Source: CAD feature listing. Evaluate the final solid. Frame: model axes, mm. A direction names the side the tool comes from. Round coordinates to 2 decimals unless told otherwise and drop trailing zeros. Loops run counter-clockwise (first coordinate to the right, second up) from the corner with the lowest first, then second, coordinate; pieces in that order, holes last.
(1) Section B-B, the plane x = -13. Return the cut outline in (y, z), plus the area to 3 significant figures.
(2) Set-up query: faces 1 (the flat face through (-29.5, -1.2, 1.2)), 2 (the flat face through (0, -4, -14)), 3 (the cylindrical face through (67.744, 19.334, -2.539)), 4 (the cylindrical face through (4.51, 6.31, -20.03)), 5 (the cylindrical face through (-27.5, 6.8, 0)). Return all of +Z, -Z, +X, -X, +Y, -Y with unobstructed straight access to the full face (end or side cutting, diameter ignored); none if empty.
(3) Section A-A, the plane x = 41.5. Return the cut outline in (y, z), plus the area to 3 significant figures.
(4) First-contact query: pin 1 Ø2 at (y, z) = (17.5, 0) entering from -X; pin 2 Ø12 at (x, y) = (-11, -5) entering from -Z; pin 3 Ø8 at (x, z) = (-19, -0.5) entering from -Y. Flat tips, straight axial feed; report the tip coordinate or a pass-through.
(5) Mould query, pull axis Z, two halves, no side actions, for faces 6 (the cylindrical face through (3.042, 0.496, -19.074)), 7 (the cylindrical face through (-3.493, 6.645, -0.251)), 8 (the cylindrical face through (3.04, 18.89, -0.89)), 9 (the flat face through (-18, 7, 2)). Classes: pulls with the +Z half, pulls with the -Z half, needs draft (parallel to the pull), parting line crosses it, or undercut.
(6) Material intervals for probe 1 along Y at (x, z) = (-28, 0) (3 decimals); probe 2 along Y at (x, z) = (67.4, 0), sorted ascending.
```python
from build123d import *

# Parameters (mm, degrees)
SKETCH2_R                = 14
BOSS_EXTRUDE1_DEPTH      = 3
SKETCH3_R                = 6
BOSS_EXTRUDE2_DEPTH      = 26.5
BOSS_EXTRUDE3_DEPTH      = 1
BOSS_EXTRUDE4_REACH      = 80.626
BOSS_EXTRUDE4_END_RADIUS = 6
HOLE1_D                  = 39
HOLE1_DEPTH              = 4.45
HOLE2_D                  = 3.3
HOLE2_DEPTH              = 6
HOLE2_TIP                = 0.991420021
HOLE3_D                  = 3.3
HOLE3_DEPTH              = 6
HOLE3_TIP                = 0.991420021
HOLE4_D                  = 3.3
HOLE4_DEPTH              = 6
HOLE4_TIP                = 0.991420021
HOLE5_D                  = 3.3
HOLE5_DEPTH              = 6
HOLE5_TIP                = 0.991420021
HOLE6_D                  = 1.25
HOLE6_DEPTH              = 1.939156082
HOLE6_CSINK_D            = 2.65
HOLE6_CSINK_ANGLE        = 60
HOLE6_TIP                = 0.360843918


with BuildPart() as part:
    # Sketch1 → Revolve1 (revolve)
    with BuildSketch(Plane.XY, mode=Mode.PRIVATE) as revolve1_sk:
        with BuildLine():
            Line((0, 21), (0, 0))
            Line((0, 0), (70, 0))
            Line((70, 0), (70, 21))
            Line((70, 21), (9.25, 21))
            ThreePointArc((9.25, 21), (9.2, 20.98660254), (9.15, 21))
            Line((9.15, 21), (0, 21))
        make_face()
    revolve(revolve1_sk.sketch.rotate(Axis((0, 0, 0), (1, 0, 0)), 270), axis=Axis((0, 0, 0), (1, 0, 0)))

    # Sketch2 → Boss-Extrude1 (add)
    with BuildSketch(Plane.ZY):
        Circle(SKETCH2_R)
    extrude(amount=BOSS_EXTRUDE1_DEPTH)

    # Sketch3 → Boss-Extrude2 (add)
    with BuildSketch(Plane.ZY.offset(3)):
        Circle(SKETCH3_R)
    extrude(amount=BOSS_EXTRUDE2_DEPTH)

    # Sketch4 → Boss-Extrude3 (add)
    with BuildSketch(Plane.ZY.offset(3)):
        with BuildLine():
            Line((0.293916284, -7.616838781), (0.293916284, -5.992796778))
            ThreePointArc((0.293916284, -5.992796778), (0, 6), (-0.293916284, -5.992796778))
            Line((-0.293916284, -5.992796778), (-0.293916284, -7.616838781))
            ThreePointArc((-0.293916284, -7.616838781), (-1.755912185, -7.072113956), (-2.882513969, -5.992796778))
            ThreePointArc((-2.882513969, -5.992796778), (0, 6.65), (2.882513969, -5.992796778))
            ThreePointArc((2.882513969, -5.992796778), (1.821852016, -7.17721696), (0.293916284, -7.616838781))
        make_face()
    extrude(amount=BOSS_EXTRUDE3_DEPTH)

    # Boss-Extrude4: up to this cylinder (the profile starts outside it)
    boss_extrude4_end = Plane(origin=(-17.5, 0, 0), z_dir=(1, 0, 0)) * Cylinder(BOSS_EXTRUDE4_END_RADIUS, 174.252, mode=Mode.PRIVATE)
    # Sketch5 → Boss-Extrude4 (add, up to the surface)
    with BuildSketch(Plane(origin=(0, 8, 0), x_dir=(-1, 0, 0), z_dir=(0, 1, 0)), mode=Mode.PRIVATE) as boss_extrude4_sk1:
        with BuildLine():
            Line((9.5, -2), (25.5, -2))
            ThreePointArc((25.5, -2), (27.5, 0), (25.5, 2))
            Line((25.5, 2), (9.5, 2))
            ThreePointArc((9.5, 2), (7.5, 0), (9.5, -2))
        make_face()
    boss_extrude4_tool1 = extrude(boss_extrude4_sk1.sketch, amount=-BOSS_EXTRUDE4_REACH, mode=Mode.PRIVATE) - boss_extrude4_end
    add(boss_extrude4_tool1.solids().sort_by_distance((-17.5, 8, 0))[0])

    # Hole1
    with Locations(Plane(origin=(70, 0, 0), x_dir=(0, 0, -1), z_dir=(1, 0, 0))):
        with Locations((0, 0)):
            Hole(HOLE1_D / 2, depth=HOLE1_DEPTH)

    # Hole2
    with Locations(Plane.ZY):
        with Locations((-17.5, 3.0543e-05)):
            Hole(HOLE2_D / 2, depth=HOLE2_DEPTH)
            with Locations((0, 0, -(HOLE2_DEPTH + HOLE2_TIP / 2))):  # 118° drill point
                Cone(0, HOLE2_D / 2, HOLE2_TIP, mode=Mode.SUBTRACT)

    # Hole3
    with Locations(Plane.ZY):
        with Locations((-3.0543e-05, -17.5)):
            Hole(HOLE3_D / 2, depth=HOLE3_DEPTH)
            with Locations((0, 0, -(HOLE3_DEPTH + HOLE3_TIP / 2))):  # 118° drill point
                Cone(0, HOLE3_D / 2, HOLE3_TIP, mode=Mode.SUBTRACT)

    # Hole4
    with Locations(Plane.ZY):
        with Locations((17.5, -3.0543e-05)):
            Hole(HOLE4_D / 2, depth=HOLE4_DEPTH)
            with Locations((0, 0, -(HOLE4_DEPTH + HOLE4_TIP / 2))):  # 118° drill point
                Cone(0, HOLE4_D / 2, HOLE4_TIP, mode=Mode.SUBTRACT)

    # Hole5
    with Locations(Plane.ZY):
        with Locations((3.0543e-05, 17.5)):
            Hole(HOLE5_D / 2, depth=HOLE5_DEPTH)
            with Locations((0, 0, -(HOLE5_DEPTH + HOLE5_TIP / 2))):  # 118° drill point
                Cone(0, HOLE5_D / 2, HOLE5_TIP, mode=Mode.SUBTRACT)

    # Hole6
    with Locations(Plane.ZY.offset(29.5)):
        with Locations((0, 0)):
            CounterSinkHole(HOLE6_D / 2, HOLE6_CSINK_D / 2, depth=HOLE6_DEPTH, counter_sink_angle=HOLE6_CSINK_ANGLE)
            with Locations((0, 0, -(HOLE6_DEPTH + HOLE6_TIP / 2))):  # 120° drill point
                Cone(0, HOLE6_D / 2, HOLE6_TIP, mode=Mode.SUBTRACT)


solid = part.part
```
Output values:
1. outline: (5.66, -2) - (8, -2) - (8, 2) - (5.66, 2) arc R6 ccw (long way) to start
1. area: 122 mm2
2. face 1: +Z, -Z, -X, +Y, -Y
2. face 2: -X
2. face 3: +X
2. face 4: +X, -X
2. face 5: -X, +Y
3. outline: circle Ø42 at (0, 0)
3. area: 1,390 mm2
4. pin 1: stops at x = 6.39
4. pin 2: stops at z = -6
4. pin 3: stops at y = -6
5. face 6: undercut
5. face 7: parting line crosses it
5. face 8: undercut
5. face 9: pulls with the +Z half
6. probe 1: y = -6 to -0.625, 0.625 to 6
6. probe 2: y = -21 to -19.5, 19.5 to 21
